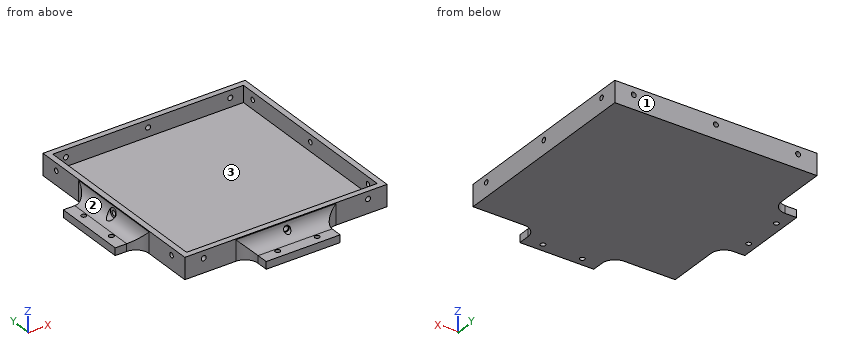
from build123d import *

# Parameters (mm, degrees)
SKETCH_3_W               = 123
SKETCH_3_H               = 123
EXTRUDE_2_DEPTH          = 3
SKETCH_4_W               = 123
SKETCH_4_H               = 123
SKETCH_4_W_2             = 116
SKETCH_4_H_2             = 116
EXTRUDE_3_DEPTH          = 10
SKETCH_7_R               = 1.5
CUT_EXTRUDE_1_DEPTH      = 139.131278138
SKETCH_9_R               = 1.5
CUT_EXTRUDE_2_DEPTH      = 139.131278138
SKETCH_10_W              = 45
SKETCH_10_H              = 15
EXTRUDE_4_DEPTH          = 4.5
SKETCH_11_R              = 1.5
CUT_EXTRUDE_3_DEPTH      = 99.522839992
PATTERN_CIRCULAR_1_COUNT = 2
PATTERN_CIRCULAR_1_ANGLE = 90
FILLET_1_R               = 8
SKETCH_13_R              = 3
CUT_EXTRUDE_4_DEPTH      = 146.431255238
SKETCH_14_R              = 2.049164466
CUT_EXTRUDE_6_DEPTH      = 146.431255238


with BuildPart() as part:
    # 草图3 → 凸台-拉伸2 (new body)
    with BuildSketch(Plane.XY):
        Rectangle(SKETCH_3_W, SKETCH_3_H)
    extrude(amount=EXTRUDE_2_DEPTH)

    # 草图4 → 凸台-拉伸3 (add)
    with BuildSketch(Plane.XY.offset(3)):
        Rectangle(SKETCH_4_W, SKETCH_4_H)
        Rectangle(SKETCH_4_W_2, SKETCH_4_H_2, mode=Mode.SUBTRACT)
    extrude(amount=EXTRUDE_3_DEPTH)

    # 草图7 → 切除-拉伸1 (cut, through all)
    with BuildSketch(Plane.XZ.offset(61.5)):
        with Locations((0, 8.5)):
            Circle(SKETCH_7_R)
        with Locations((50, 8.5)):
            Circle(SKETCH_7_R)
        with Locations((-50, 8.5)):
            Circle(SKETCH_7_R)
    extrude(amount=-CUT_EXTRUDE_1_DEPTH, mode=Mode.SUBTRACT)

    # 草图9 → 切除-拉伸2 (cut, through all)
    with BuildSketch(Plane.ZY.offset(61.5)):
        with Locations((8.5, 0)):
            Circle(SKETCH_9_R)
        with Locations((8.5, -50)):
            Circle(SKETCH_9_R)
        with Locations((8.5, 50)):
            Circle(SKETCH_9_R)
    extrude(amount=-CUT_EXTRUDE_2_DEPTH, mode=Mode.SUBTRACT)

    # 草图10 → 凸台-拉伸4 (add)
    with BuildSketch(Plane(origin=(0, 0, 0), x_dir=(-1, 0, 0), z_dir=(0, 0, -1))):
        with Locations((0, -69)):
            Rectangle(SKETCH_10_W, SKETCH_10_H)
    extrude_4 = extrude(amount=-EXTRUDE_4_DEPTH)

    # 草图11 → 切除-拉伸3 (cut, through all)
    with BuildSketch(Plane.XY.offset(4.5)):
        with Locations((-12, -71.5)):
            Circle(SKETCH_11_R)
        with Locations((12, -71.5)):
            Circle(SKETCH_11_R)
    cut_extrude_3 = extrude(amount=-CUT_EXTRUDE_3_DEPTH, mode=Mode.SUBTRACT)

    # 阵列(圆周)1: 凸台-拉伸4, 切除-拉伸3 ×2 about axis
    pattern_circular_1_axis = Axis((0, 0, 0), (0, 0, -1))
    add([extrude_4.rotate(pattern_circular_1_axis, i * PATTERN_CIRCULAR_1_ANGLE / (PATTERN_CIRCULAR_1_COUNT - 1)) for i in range(1, PATTERN_CIRCULAR_1_COUNT)])
    add([cut_extrude_3.rotate(pattern_circular_1_axis, i * PATTERN_CIRCULAR_1_ANGLE / (PATTERN_CIRCULAR_1_COUNT - 1)) for i in range(1, PATTERN_CIRCULAR_1_COUNT)], mode=Mode.SUBTRACT)

    # 圆角1
    # the kernel refuses this fillet: 8 mm, written as the material it adds along each edge
    with BuildSketch(Plane(origin=(-61.5, 22.5, 0), x_dir=(0, 1, 0), z_dir=(0, 0, 1)), Plane(origin=(-22.5, -61.5, 0), x_dir=(-1, 0, 0), z_dir=(0, 0, 1))) as fillet_1_piece_1:
        with BuildLine():
            CenterArc((FILLET_1_R, FILLET_1_R), FILLET_1_R, 180, 90)
            Line((0, FILLET_1_R), (0, 0))
            Line((0, 0), (FILLET_1_R, 0))
        make_face()
    extrude(amount=4.5)
    with BuildSketch(Plane(origin=(-61.5, -22.5, 4.5), x_dir=(0, 0, 1), z_dir=(0, 1, 0))) as fillet_1_piece_2_section:
        with BuildLine():
            CenterArc((FILLET_1_R, -FILLET_1_R), FILLET_1_R, 90, 90)
            Line((0, -FILLET_1_R), (0, 0))
            Line((0, 0), (FILLET_1_R, 0))
        make_face()
    fillet_1_piece_2 = extrude(amount=45, mode=Mode.PRIVATE)
    fillet_1_piece_2 = fillet_1_piece_2 - Plane(origin=(-63.326853287, 0, 8.5), x_dir=(0, 0, 1), z_dir=(-1, 0, 0)) * Cylinder(1.5, 122, mode=Mode.PRIVATE)
    add(fillet_1_piece_2)
    with BuildSketch(Plane(origin=(-61.5, -22.5, 0), x_dir=(0, -1, 0), z_dir=(0, 0, 1)), Plane(origin=(22.5, -61.5, 0), x_dir=(1, 0, 0), z_dir=(0, 0, 1))) as fillet_1_piece_3:
        with BuildLine():
            CenterArc((FILLET_1_R, -FILLET_1_R), FILLET_1_R, 90, 90)
            Line((0, -FILLET_1_R), (0, 0))
            Line((0, 0), (FILLET_1_R, 0))
        make_face()
    extrude(amount=4.5)
    with BuildSketch(Plane(origin=(22.5, -61.5, 4.5), x_dir=(0, 0, 1), z_dir=(-1, 0, 0))) as fillet_1_piece_4_section:
        with BuildLine():
            CenterArc((FILLET_1_R, -FILLET_1_R), FILLET_1_R, 90, 90)
            Line((0, -FILLET_1_R), (0, 0))
            Line((0, 0), (FILLET_1_R, 0))
        make_face()
    fillet_1_piece_4 = extrude(amount=45, mode=Mode.PRIVATE)
    fillet_1_piece_4 = fillet_1_piece_4 - Plane(origin=(0, -63.326852549, 8.5), x_dir=(1, 0, 0), z_dir=(0, -1, 0)) * Cylinder(1.5, 122, mode=Mode.PRIVATE)
    add(fillet_1_piece_4)
    with BuildSketch(Plane(origin=(-61.5, -22.5, 4.5), x_dir=(0, 0, 1), z_dir=(0, 1, 0))) as fillet_1_piece_5a_section:
        with BuildLine():
            CenterArc((FILLET_1_R, -FILLET_1_R), FILLET_1_R, 90, 90)
            Line((0, -FILLET_1_R), (0, 0))
            Line((0, 0), (FILLET_1_R, 0))
        make_face()
    fillet_1_piece_5a = extrude(amount=65, mode=Mode.PRIVATE)
    fillet_1_piece_5a = split(fillet_1_piece_5a, bisect_by=Plane(origin=(-63.311160914, 22.5, 6.311160914), z_dir=(0, 1, 0)), keep=Keep.TOP, mode=Mode.PRIVATE)
    with BuildSketch(Plane(origin=(-61.5, 22.5, 0), x_dir=(0, 1, 0), z_dir=(0, 0, 1))) as fillet_1_piece_5b_section:
        with BuildLine():
            CenterArc((FILLET_1_R, FILLET_1_R), FILLET_1_R, 180, 90)
            Line((0, FILLET_1_R), (0, 0))
            Line((0, 0), (FILLET_1_R, 0))
        make_face()
    fillet_1_piece_5b = extrude(amount=24.5, mode=Mode.PRIVATE)
    fillet_1_piece_5b = split(fillet_1_piece_5b, bisect_by=Plane(origin=(-63.311160914, 24.311160914, 13), z_dir=(0, 0, -1)), keep=Keep.TOP, mode=Mode.PRIVATE)
    fillet_1_piece_5b = split(fillet_1_piece_5b, bisect_by=Plane(origin=(-63.311160914, 24.311160914, 4.5), z_dir=(0, 0, 1)), keep=Keep.TOP, mode=Mode.PRIVATE)
    fillet_1_piece_5 = fillet_1_piece_5a & fillet_1_piece_5b
    add(fillet_1_piece_5)
    with BuildSketch(Plane(origin=(-61.5, -22.5, 0), x_dir=(0, -1, 0), z_dir=(0, 0, 1))) as fillet_1_piece_6a_section:
        with BuildLine():
            CenterArc((FILLET_1_R, -FILLET_1_R), FILLET_1_R, 90, 90)
            Line((0, -FILLET_1_R), (0, 0))
            Line((0, 0), (FILLET_1_R, 0))
        make_face()
    fillet_1_piece_6a = extrude(amount=24.5, mode=Mode.PRIVATE)
    fillet_1_piece_6a = split(fillet_1_piece_6a, bisect_by=Plane(origin=(-63.311160914, -24.311160914, 13), z_dir=(0, 0, -1)), keep=Keep.TOP, mode=Mode.PRIVATE)
    fillet_1_piece_6a = split(fillet_1_piece_6a, bisect_by=Plane(origin=(-63.311160914, -24.311160914, 4.5), z_dir=(0, 0, 1)), keep=Keep.TOP, mode=Mode.PRIVATE)
    with BuildSketch(Plane(origin=(-61.5, -42.5, 4.5), x_dir=(0, 0, 1), z_dir=(0, 1, 0))) as fillet_1_piece_6b_section:
        with BuildLine():
            CenterArc((FILLET_1_R, -FILLET_1_R), FILLET_1_R, 90, 90)
            Line((0, -FILLET_1_R), (0, 0))
            Line((0, 0), (FILLET_1_R, 0))
        make_face()
    fillet_1_piece_6b = extrude(amount=65, mode=Mode.PRIVATE)
    fillet_1_piece_6b = split(fillet_1_piece_6b, bisect_by=Plane(origin=(-63.311160914, -22.5, 6.311160914), z_dir=(0, -1, 0)), keep=Keep.TOP, mode=Mode.PRIVATE)
    fillet_1_piece_6 = fillet_1_piece_6a & fillet_1_piece_6b
    add(fillet_1_piece_6)
    with BuildSketch(Plane(origin=(22.5, -61.5, 4.5), x_dir=(0, 0, 1), z_dir=(-1, 0, 0))) as fillet_1_piece_7a_section:
        with BuildLine():
            CenterArc((FILLET_1_R, -FILLET_1_R), FILLET_1_R, 90, 90)
            Line((0, -FILLET_1_R), (0, 0))
            Line((0, 0), (FILLET_1_R, 0))
        make_face()
    fillet_1_piece_7a = extrude(amount=65, mode=Mode.PRIVATE)
    fillet_1_piece_7a = split(fillet_1_piece_7a, bisect_by=Plane(origin=(-22.5, -63.311160914, 6.311160914), z_dir=(-1, 0, 0)), keep=Keep.TOP, mode=Mode.PRIVATE)
    with BuildSketch(Plane(origin=(-22.5, -61.5, 0), x_dir=(-1, 0, 0), z_dir=(0, 0, 1))) as fillet_1_piece_7b_section:
        with BuildLine():
            CenterArc((FILLET_1_R, FILLET_1_R), FILLET_1_R, 180, 90)
            Line((0, FILLET_1_R), (0, 0))
            Line((0, 0), (FILLET_1_R, 0))
        make_face()
    fillet_1_piece_7b = extrude(amount=24.5, mode=Mode.PRIVATE)
    fillet_1_piece_7b = split(fillet_1_piece_7b, bisect_by=Plane(origin=(-24.311160914, -63.311160914, 13), z_dir=(0, 0, -1)), keep=Keep.TOP, mode=Mode.PRIVATE)
    fillet_1_piece_7b = split(fillet_1_piece_7b, bisect_by=Plane(origin=(-24.311160914, -63.311160914, 4.5), z_dir=(0, 0, 1)), keep=Keep.TOP, mode=Mode.PRIVATE)
    fillet_1_piece_7 = fillet_1_piece_7a & fillet_1_piece_7b
    add(fillet_1_piece_7)
    with BuildSketch(Plane(origin=(22.5, -61.5, 0), x_dir=(1, 0, 0), z_dir=(0, 0, 1))) as fillet_1_piece_8a_section:
        with BuildLine():
            CenterArc((FILLET_1_R, -FILLET_1_R), FILLET_1_R, 90, 90)
            Line((0, -FILLET_1_R), (0, 0))
            Line((0, 0), (FILLET_1_R, 0))
        make_face()
    fillet_1_piece_8a = extrude(amount=24.5, mode=Mode.PRIVATE)
    fillet_1_piece_8a = split(fillet_1_piece_8a, bisect_by=Plane(origin=(24.311160914, -63.311160914, 13), z_dir=(0, 0, -1)), keep=Keep.TOP, mode=Mode.PRIVATE)
    fillet_1_piece_8a = split(fillet_1_piece_8a, bisect_by=Plane(origin=(24.311160914, -63.311160914, 4.5), z_dir=(0, 0, 1)), keep=Keep.TOP, mode=Mode.PRIVATE)
    with BuildSketch(Plane(origin=(42.5, -61.5, 4.5), x_dir=(0, 0, 1), z_dir=(-1, 0, 0))) as fillet_1_piece_8b_section:
        with BuildLine():
            CenterArc((FILLET_1_R, -FILLET_1_R), FILLET_1_R, 90, 90)
            Line((0, -FILLET_1_R), (0, 0))
            Line((0, 0), (FILLET_1_R, 0))
        make_face()
    fillet_1_piece_8b = extrude(amount=65, mode=Mode.PRIVATE)
    fillet_1_piece_8b = split(fillet_1_piece_8b, bisect_by=Plane(origin=(22.5, -63.311160914, 6.311160914), z_dir=(1, 0, 0)), keep=Keep.TOP, mode=Mode.PRIVATE)
    fillet_1_piece_8 = fillet_1_piece_8a & fillet_1_piece_8b
    add(fillet_1_piece_8)

    # 草图13 → 切除-拉伸4 (cut, through all)
    with BuildSketch(Plane.ZY.offset(61.5)):
        with Locations(Location((8.5, 0, 0), (0, 0, 180))):
            Circle(SKETCH_13_R)
    extrude(amount=CUT_EXTRUDE_4_DEPTH, mode=Mode.SUBTRACT)

    # 草图14 → 切除-拉伸6 (cut, through all)
    with BuildSketch(Plane.XZ.offset(61.5)):
        with Locations(Location((0, 8.5, 0), (0, 0, 180))):
            Circle(SKETCH_14_R)
    extrude(amount=CUT_EXTRUDE_6_DEPTH, mode=Mode.SUBTRACT)


solid = part.part
Check sheet for the modelled part. Datum: model origin and axes. Units: mm. Face numbers are marked on the shaded views. Give positions to 0.01 mm unless a question says otherwise; leave off trailing zeros. Write each loop counter-clockwise with the first axis right and the second up, starting at its lowest first coordinate (ties: lowest second). Pieces come first, ordered by that corner, then holes. Notation, with made-up numbers: (17, 45) -> (25, 45) arc R27 ccw to (25, 78) -> close; hole circle Ø9 at (-19, -37). An arc over 180 degrees is marked (long way). Use one line per item in the form item = value. Start each with the question number.
1. Section check A-A (x = 8). Record the cut outline in (y, z).
2. Go/stop test with flat-tipped pins: P1, Ø4, axis at x = -71.5, y = 12, coming from the +Z side; P2, Ø12, axis at x = 19, y = 24, coming from the +Z side; P3, Ø1.8, axis at x = 50, z = 8.5, coming from the -Y side; P4, Ø5, axis at x = -73, z = 2.5, coming from the +Y side. Record where each tip stops, or that it passes through.
3. Mould release check, pull along Y, two halves, no side actions. Record for the marked faces 1, 2 and 3: pulls with the +Y half, pulls with the -Y half, needs draft (parallel to the pull), parting line crosses it, or undercut.
4. Thickness scan on line 1 along Y through (x, z) = (58.9, 8.5); line 2 along Y through (x, z) = (-52, 5); line 3 along X through (y, z) = (9.5, 4). Record the ranges inside material, lowest first. Write a range as from..to.
Conclusion:
q1.outline = (-76.5, 0) -> (61.5, 0) -> (61.5, 13) -> (58, 13) -> (58, 3) -> (-58, 3) -> (-58, 13) -> (-61.5, 13) -> (-61.5, 12.5) arc R8 cw to (-69.5, 4.5) -> (-76.5, 4.5) -> close
q2.P1 = 4.5
q2.P2 = 3
q2.P3 = through
q2.P4 = 22.5
q3.face_1 = pulls with the +Y half
q3.face_2 = needs draft
q3.face_3 = undercut
q4.line_1 = -61.5..-51.5, -48.5..-1.5, 1.5..48.5, 51.5..61.5
q4.line_2 = -61.5..-58, 58..61.5
q4.line_3 = -76.5..-58, 58..61.5
